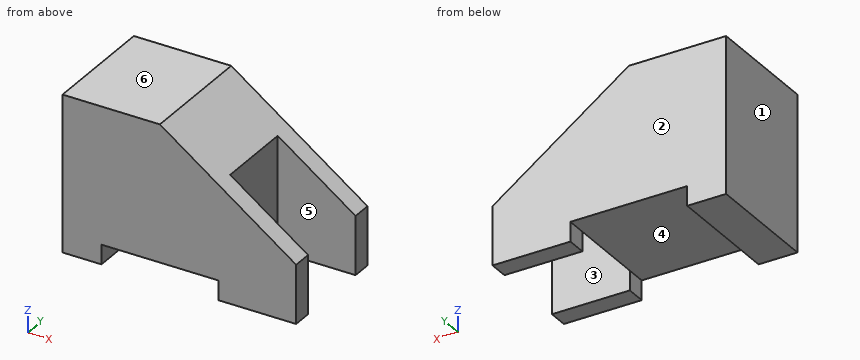
from build123d import *

# Parameters (mm, degrees)
F0_W     = 60
F0_H     = 40
F1_DEPTH = 30
F2_W     = 30
F2_H     = 5
F3_DEPTH = 30.001
F5_W     = 20
F5_H     = 30
F6_DEPTH = 20


with BuildPart() as f1:
    # F0 (on Front) → F1 (new body)
    with BuildSketch(Plane.XZ):
        with Locations((30, 20)):
            Rectangle(F0_W, F0_H)
    extrude(amount=-F1_DEPTH)

    # F2 (on face) → F3 (cut, through all)
    with BuildSketch(Plane.XZ):
        with Locations((25, 2.5)):
            Rectangle(F2_W, F2_H)
        Polygon((60, 40), (25, 40), (60, 15), align=None)
    extrude(amount=-F3_DEPTH, mode=Mode.SUBTRACT)

    # F5 (on offset) → F6 (cut)
    with BuildSketch(Plane.YZ.offset(60)):
        with Locations((15, 15)):
            Rectangle(F5_W, F5_H)
    extrude(amount=-F6_DEPTH, mode=Mode.SUBTRACT)


solid = f1.part
Model file for the job. Use its own axes, mm. Face numbers are marked on the shaded views. A direction names the side the tool comes from. Give positions to 0.01 mm unless a question says otherwise; leave off trailing zeros. Loops run counter-clockwise (first coordinate to the right, second up) from the corner with the lowest first, then second, coordinate; pieces in that order, holes last.
Item 1: Slice it at B-B (x = 51.5). Write the cut outline in (y, z).
Check values:
outline: (0, 0) - (5, 0) - (5, 21.07) - (0, 21.07) - close; (25, 0) - (30, 0) - (30, 21.07) - (25, 21.07) - close
Item 2: Slice it at A-A (z = 3). Write the cut outline in (x, y).
Check values:
outline: (0, 0) - (10, 0) - (10, 30) - (0, 30) - close; (40, 0) - (60, 0) - (60, 5) - (40, 5) - close; (40, 25) - (60, 25) - (60, 30) - (40, 30) - close
Item 3: Mould opens along Y. For the marked faces 1, 2 and 3 say: +Y half, -Y half, draft (parallel to the pull), parting line (faces both ways), or undercut.
Check values:
face 1: draft
face 2: +Y half
face 3: undercut
Item 4: Drill centre lines: line 1 along Y through (x, z) = (57.5, 5); line 2 along X through (y, z) = (4.75, 3); line 3 along Z through (x, y) = (22, 13). Where is each one in solid material? Low to high.
Check values:
line 1: y = 0 to 5, 25 to 30
line 2: x = 0 to 10, 40 to 60
line 3: z = 5 to 40
Item 5: Which spindle directions (+Z, -Z, +X, -X, +Y, -Y) get a long thin tool onto all of the face, cutting with end or side? Do the marked faces 4, 5 and 6. Say none if no direction does.
Check values:
face 4: -Z, +Y, -Y
face 5: +Z, -Z, +X
face 6: +Z, +X, -X, +Y, -Y
Item 6: Slice it at C-C (y = 26.5). Write the cut outline in (x, z).
Check values:
outline: (0, 0) - (10, 0) - (10, 5) - (40, 5) - (40, 0) - (60, 0) - (60, 15) - (25, 40) - (0, 40) - close
Item 7: Drop flat-ended pins along their axis: P1, Ø1, axis at y = 26, z = 19, coming from the +X side; P2, Ø5.5, axis at y = 12.5, z = 3.5, coming from the +X side; P3, Ø1.5, axis at x = 40, y = 7, coming from the -Z side. Give the stop position or say it passes through.
Check values:
P1: stops at x = 55.1
P2: stops at x = 40
P3: stops at z = 5
Item 8: Slice it at D-D (z = 13). Write the cut outline in (x, y), plus the area to 3 significant figures.
Check values:
outline: (0, 0) - (60, 0) - (60, 5) - (40, 5) - (40, 25) - (60, 25) - (60, 30) - (0, 30) - close
area: 1,400 mm2
